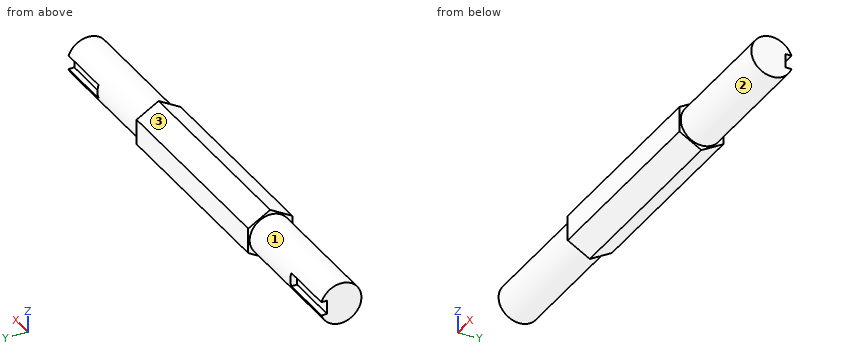
from build123d import *

# Parameters (mm, degrees)
SKETCH1_R           = 15
BOSS_EXTRUDE2_DEPTH = 168.7
BOSS_EXTRUDE3_DEPTH = 74.5
SKETCH3_W           = 10
SKETCH3_H           = 10
CUT_EXTRUDE1_DEPTH  = 40


with BuildPart() as part:
    # Sketch1 → Boss-Extrude2 (new, symmetric)
    with BuildSketch(Plane(origin=(0, 0, 0), x_dir=(0, 0, -1), z_dir=(1, 0, 0))):
        Circle(SKETCH1_R)
    extrude(amount=BOSS_EXTRUDE2_DEPTH, both=True)

    # Sketch2 → Boss-Extrude3 (add, symmetric)
    with BuildSketch(Plane(origin=(0, 0, 0), x_dir=(0, 0, -1), z_dir=(1, 0, 0))):
        Polygon((-18.504076128, 0), (-9.252038064, -16.025), (9.252038064, -16.025), (18.504076128, 0), (9.252038064, 16.025), (-9.252038064, 16.025), align=None)
    extrude(amount=BOSS_EXTRUDE3_DEPTH, both=True)

    # Sketch3 → Cut-Extrude1 (cut)
    with BuildSketch(Plane(origin=(168.7, 0, 0), x_dir=(0, 0, -1), z_dir=(1, 0, 0))):
        with Locations((0, 15)):
            Rectangle(SKETCH3_W, SKETCH3_H)
    cut_extrude1 = extrude(amount=-CUT_EXTRUDE1_DEPTH, mode=Mode.SUBTRACT)

    # Mirror1: Cut-Extrude1 across plane
    add(cut_extrude1.mirror(Plane(origin=(0, 0, 0), x_dir=(0, 0, 1), z_dir=(1, 0, 0))), mode=Mode.SUBTRACT)


solid = part.part
Read the model definition and answer for the solid it produces. Units are mm, in the model's axes. Face numbers are marked on the shaded views. A direction names the side the tool comes from. Round coordinates to 2 decimals unless told otherwise and drop trailing zeros. Loops run counter-clockwise (first coordinate to the right, second up) from the corner with the lowest first, then second, coordinate; pieces in that order, holes last.
Q1. Section B-B on x = -22 is taken. Write down the section's boundary in (y, z) (3 decimals), and give its area (3 significant figures).
Q2. Which of the six approach directions +Z, -Z, +X, -X, +Y, -Y give full straight-line access (tool end or side, diameter ignored) to the marked faces 1, 2 and 3?
Q3. Each of these flat-tipped pins is pushed along its axis until it touches: pin 1 (4.5 mm diameter, centred on x = 150, y = 13, fed in from -Z); pin 2 (1.5 mm diameter, centred on y = 12.5, z = 2, fed in from -X); pin 3 (8 mm diameter, centred on x = -149, z = -1.5, fed in from +Y). Where does it stop, or does it pass through?
Q4. Consider probe 1 along X at (y, z) = (15.5, 2); probe 2 along Z at (x, y) = (-58, -6); probe 3 along X at (y, z) = (14, 3). Determine where each line is inside the solid, lowest interval first.
Q5. Section C-C on y = -12 is taken. Write down the section's boundary in (x, z), and give its area (3 significant figures).
Q6. Section A-A on z = 0 is taken. Write down the section's boundary in (x, y) (3 decimals), and give its area (3 significant figures).
Q7. Section D-D on x = -115.5 is taken. Write down the section's boundary in (y, z), and give its area (3 significant figures).
Output:
1. outline: (-16.025, -9.252) - (0, -18.504) - (16.025, -9.252) - (16.025, 9.252) - (0, 18.504) - (-16.025, 9.252) - close
1. area: 890 mm2
2. face 1: -X
2. face 2: +X
2. face 3: +Z, +X, -X, +Y
3. pin 1: stops at z = -10.46
3. pin 2: stops at x = -128.7
3. pin 3: stops at y = 14.14
4. probe 1: x = -74.5 to 74.5
4. probe 2: z = -15.04 to 15.04
4. probe 3: x = -128.7 to 128.7
5. outline: (-168.7, -9) - (-74.5, -9) - (-74.5, -11.58) - (74.5, -11.58) - (74.5, -9) - (168.7, -9) - (168.7, 9) - (74.5, 9) - (74.5, 11.58) - (-74.5, 11.58) - (-74.5, 9) - (-168.7, 9) - close
5. area: 6,840 mm2
6. outline: (-168.7, -15) - (-74.5, -15) - (-74.5, -16.025) - (74.5, -16.025) - (74.5, -15) - (168.7, -15) - (168.7, 10) - (128.7, 10) - (128.7, 15) - (74.5, 15) - (74.5, 16.025) - (-74.5, 16.025) - (-74.5, 15) - (-128.7, 15) - (-128.7, 10) - (-168.7, 10) - close
6. area: 10,000 mm2
7. outline: circle Ø30 at (0, 0)
7. area: 707 mm2
